Could you check a few things on this model? Use its own coordinates, in mm. Face numbers are marked on the shaded views. A direction names the side the tool comes from. Give positions to 0.01 mm unless a question says otherwise; leave off trailing zeros. Write each loop counter-clockwise with the first axis right and the second up, starting at its lowest first coordinate (ties: lowest second). Pieces come first, ordered by that corner, then holes. Notation, with made-up numbers: (11.25, 57.5) - (58.25, 57.5) arc R24 cw to (58.25, 74.5) - close; hole circle Ø2 at (11.25, 76). An arc over 180 degrees is marked (long way). Answer in a Markdown table with one row per item.
from build123d import *

# Parameters (mm, degrees)
SKETCH3_W           = 90
SKETCH3_H           = 90
BOSS_EXTRUDE1_DEPTH = 350
SHELL1_T            = -5
SKETCH4_W           = 100
SKETCH4_H           = 50
CUT_EXTRUDE1_DEPTH  = 20
SKETCH5_W           = 100
SKETCH5_H           = 100
SKETCH5_W_2         = 90
SKETCH5_H_2         = 90
BOSS_EXTRUDE2_DEPTH = 5
SKETCH6_W           = 100
SKETCH6_H           = 100
SKETCH6_W_2         = 90
SKETCH6_H_2         = 90
BOSS_EXTRUDE3_DEPTH = 5


with BuildPart() as part:
    # Sketch3 → Boss-Extrude1 (new body)
    with BuildSketch(Plane.XY):
        Rectangle(SKETCH3_W, SKETCH3_H)
    extrude(amount=BOSS_EXTRUDE1_DEPTH)

    # Shell1
    shell1_openings = [part.faces().sort_by_distance(p)[0] for p in [
        (0, 0, 350),
        (0, 0, 0),
    ]]
    offset(amount=SHELL1_T, openings=shell1_openings, kind=Kind.INTERSECTION)

    # Sketch4 → Cut-Extrude1 (cut)
    with BuildSketch(Plane(origin=(45, 0, 0), x_dir=(0, 0, -1), z_dir=(1, 0, 0))):
        with Locations((-175, 0)):
            Rectangle(SKETCH4_W, SKETCH4_H)
    extrude(amount=-CUT_EXTRUDE1_DEPTH, mode=Mode.SUBTRACT)

    # Sketch5 → Boss-Extrude2 (add)
    with BuildSketch(Plane.XY.offset(350)):
        Rectangle(SKETCH5_W, SKETCH5_H)
        Rectangle(SKETCH5_W_2, SKETCH5_H_2, mode=Mode.SUBTRACT)
    extrude(amount=-BOSS_EXTRUDE2_DEPTH)

    # Sketch6 → Boss-Extrude3 (add)
    with BuildSketch(Plane(origin=(0, 0, 0), x_dir=(-1, 0, 0), z_dir=(0, 0, -1))):
        Rectangle(SKETCH6_W, SKETCH6_H)
        Rectangle(SKETCH6_W_2, SKETCH6_H_2, mode=Mode.SUBTRACT)
    extrude(amount=-BOSS_EXTRUDE3_DEPTH)


solid = part.part
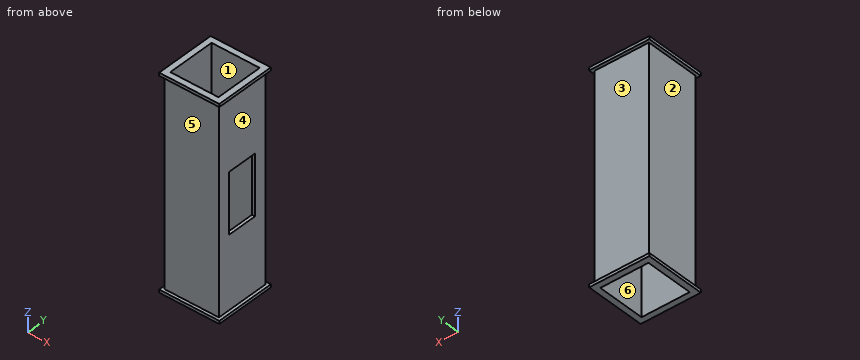
1) We'd pull the mould along Z, two halves only. Please class the marked faces 1 and 2: +Z half, -Z half, draft (parallel to the pull), parting line (faces both ways), or undercut.
Check values:
| item | result |
|---|---|
| face 1 | draft |
| face 2 | undercut |
2) If I drill on line 1 (Y direction, x = 1, z = 61.5); line 2 (X direction, y = 42, z = 201.5), over which ranges is the centre line in solid material (lowest first)?
Check values:
| item | result |
|---|---|
| line 1 | y = -45 to -40, 40 to 45 |
| line 2 | x = -45 to 45 |
3) Will these pins go through, and if not, where does the flat tip stop? P1, Ø5, axis at y = -18.5, z = 175, coming from the +X side; P2, Ø10, axis at y = 25, z = 44.5, coming from the +X side; P3, Ø8, axis at x = -34, z = 224.5, coming from the +Y side.
Check values:
| item | result |
|---|---|
| P1 | stops at x = -40 |
| P2 | stops at x = 45 |
| P3 | stops at y = 45 |
4) Imagine slicing it at A-A (z = 58). List the corners of the cut face in (x, y) for me, then the cut area to 3 significant figures.
Check values:
| item | result |
|---|---|
| outline | (-45, -45) - (45, -45) - (45, 45) - (-45, 45) - close; hole (-40, -40) - (40, -40) - (40, 40) - (-40, 40) - close |
| area | 1,700 mm2 |
5) Imagine slicing it at C-C (y = -18.5). List the corners of the cut face in (x, z) for me.
Check values:
| item | result |
|---|---|
| outline | (-50, 0) - (-40, 0) - (-40, 350) - (-50, 350) - (-50, 345) - (-45, 345) - (-45, 5) - (-50, 5) - close; (40, 0) - (50, 0) - (50, 5) - (45, 5) - (45, 125) - (40, 125) - close; (40, 225) - (45, 225) - (45, 345) - (50, 345) - (50, 350) - (40, 350) - close |
6) On a 3-axis mill with a long thin cutter (end or side, diameter ignored), from which of +Z, -Z, +X, -X, +Y, -Y can I reach the whole of each face in a straight line? I mean the marked faces 3, 4, 5 and 6. Say none if no direction works.
Check values:
| item | result |
|---|---|
| face 3 | +X, -X, +Y |
| face 4 | +X, +Y, -Y |
| face 5 | +X, -X, -Y |
| face 6 | +Z, -Z |
7) Imagine slicing it at D-D (z = 133). List the corners of the cut face in (x, y) for me, then the cut area to 3 significant figures.
Check values:
| item | result |
|---|---|
| outline | (-45, -45) - (45, -45) - (45, -25) - (40, -25) - (40, -40) - (-40, -40) - (-40, 40) - (40, 40) - (40, 25) - (45, 25) - (45, 45) - (-45, 45) - close |
| area | 1,450 mm2 |
8) Imagine slicing it at B-B (x = 5). List the corners of the cut face in (y, z) for me.
Check values:
| item | result |
|---|---|
| outline | (-50, 0) - (-40, 0) - (-40, 350) - (-50, 350) - (-50, 345) - (-45, 345) - (-45, 5) - (-50, 5) - close; (40, 0) - (50, 0) - (50, 5) - (45, 5) - (45, 345) - (50, 345) - (50, 350) - (40, 350) - close |
